```python
from build123d import *

# Parameters (mm, degrees)
SKETCH1_R           = 24
BOSS_EXTRUDE1_DEPTH = 2
SKETCH6_R           = 6.5
CUT_EXTRUDE4_DEPTH  = 2.4
SKETCH11_R          = 1.65
CUT_EXTRUDE8_DEPTH  = 35
SKETCH12_W          = 2.558537978
SKETCH12_H          = 52
BOSS_EXTRUDE2_DEPTH = 14


with BuildPart() as part:
    # Sketch1 → Boss-Extrude1 (new body)
    with BuildSketch(Plane(origin=(0, 0, 0), x_dir=(1, 0, 0), z_dir=(0, 1, 0))):
        with Locations(Location((0, 0, 0), (0, 0, 270))):
            Circle(SKETCH1_R)
    extrude(amount=BOSS_EXTRUDE1_DEPTH)

    # Sketch6 → Cut-Extrude4 (cut)
    with BuildSketch(Plane(origin=(0, 2, 0), x_dir=(1, 0, 0), z_dir=(0, 1, 0))):
        with Locations(Location((0, 0, 0), (0, 0, 270))):
            Circle(SKETCH6_R)
    extrude(amount=-CUT_EXTRUDE4_DEPTH, mode=Mode.SUBTRACT)

    # Sketch11 → Cut-Extrude8 (cut, through all)
    with BuildSketch(Plane.XZ.offset(-2)):
        with Locations(Location((16.74, 3.315, 0), (0, 0, 270))):
            Circle(SKETCH11_R)
        with Locations(Location((16.74, -3.315, 0), (0, 0, 270))):
            Circle(SKETCH11_R)
    extrude(amount=CUT_EXTRUDE8_DEPTH, mode=Mode.SUBTRACT)

    # Sketch12 → Boss-Extrude2 (add)
    with BuildSketch(Plane(origin=(0, 0, 0), x_dir=(1, 0, 0), z_dir=(0, 1, 0))):
        with Locations((-4, 0)):
            Rectangle(SKETCH12_W, SKETCH12_H)
    extrude(amount=-BOSS_EXTRUDE2_DEPTH)


solid = part.part
```
Could you check a few things on this model? Use its own coordinates, in mm. A direction names the side the tool comes from. Give positions to 0.01 mm unless a question says otherwise; leave off trailing zeros. Loops run counter-clockwise (first coordinate to the right, second up) from the corner with the lowest first, then second, coordinate; pieces in that order, holes last. Notation, with made-up numbers: (46, -28) - (102, -28) arc R18 cw to (102, -10) - close; hole circle Ø3 at (-3.75, 4.5). An arc over 180 degrees is marked (long way). Use one line per item in the form item = value.
1. I'm going to push flat-ended pins straight in: pin 1 Ø2 at (x, y) = (-1.5, -2.5) entering from -Z; pin 2 Ø1.3 at (x, z) = (-4, -24.5) entering from +Y; pin 3 Ø6 at (x, y) = (-6.5, 0) entering from -Z; pin 4 Ø4 at (y, z) = (-7, 6.5) entering from -X. Where does each tip first touch, or does it pass through?
Response values:
pin_1 = through
pin_2 = 0
pin_3 = -26
pin_4 = -5.28
2. Thinking about a two-plate mould opening in X: for faces 4 (the face through (-5.279, -7, 0)), 5 (the face through (-4, -7, 26)), 6 (the face through (18.131, 1.014, -4.202)), which applies, released by +X, released by -X, zero draft, split by the parting line, or undercut?
Response values:
face_4 = released by -X
face_5 = zero draft
face_6 = undercut
3. I want a section at D-D (z = 20.5). Please give me the cut outline in (x, y), and give its area (3 significant figures).
Response values:
outline = (-12.48, 0) - (-5.28, 0) - (-5.28, -14) - (-2.72, -14) - (-2.72, 0) - (12.48, 0) - (12.48, 2) - (-12.48, 2) - close
area = 85.7 mm²
4. I want a section at B-B (z = 0). Please give me the cut outline in (x, y).
Response values:
outline = (-24, 0) - (-6.5, 0) - (-6.5, 2) - (-24, 2) - close; (-5.28, -14) - (-2.72, -14) - (-2.72, 0) - (-5.28, 0) - close; (6.5, 0) - (24, 0) - (24, 2) - (6.5, 2) - close
5. On a 3-axis mill with a long thin cutter (end or side, diameter ignored), from which of +Z, -Z, +X, -X, +Y, -Y can I reach the whole of each face in a straight line? I mean faces 1 (the face through (-4, 0, -25)), 2 (the face through (11, 0, 0)), 3 (the face through (-4, 0, 0)). Say none if no direction works.
Response values:
face_1 = -Z, -X, +Y
face_2 = +Z, -Z, +X, -Y
face_3 = +Y
6. I need wall thicknesses on probe 1 along X at (y, z) = (1.05, 0); probe 2 along Y at (x, z) = (-16.5, 0.5). Which ranges of each line are inside material? Lowest first, please.
Response values:
probe_1 = -24 to -6.5, 6.5 to 24
probe_2 = 0 to 2
7. I want a section at C-C (x = 16.74). Please give me the cut outline in (y, z) (3 decimals).
Response values:
outline = (0, -17.198) - (2, -17.198) - (2, -4.965) - (0, -4.965) - close; (0, -1.665) - (2, -1.665) - (2, 1.665) - (0, 1.665) - close; (0, 4.965) - (2, 4.965) - (2, 17.198) - (0, 17.198) - close
8. I want a section at A-A (x = 0). Please give me the cut outline in (y, z), and give its area (3 significant figures).
Response values:
outline = (0, -24) - (2, -24) - (2, -6.5) - (0, -6.5) - close; (0, 6.5) - (2, 6.5) - (2, 24) - (0, 24) - close
area = 70.0 mm²
